CAD build for the part. Positions are in the model's coordinates, mm. Face numbers are marked on the shaded views. A direction names the side the tool comes from. Coordinates: 2 decimals unless noted, no trailing zeros. Order: outer loops, then holes, each group sorted by start corner. A loop starts at its lowest first (then second) coordinate and runs counter-clockwise, first axis right, second up. Notation, with made-up numbers: M 81.25,69.25 L 119.25,69.25 A15 ccw 119.25,96.25 Z; hole C 3.5,71.5 d9. An arc over 180 degrees is marked long. One line per item, written item: value.
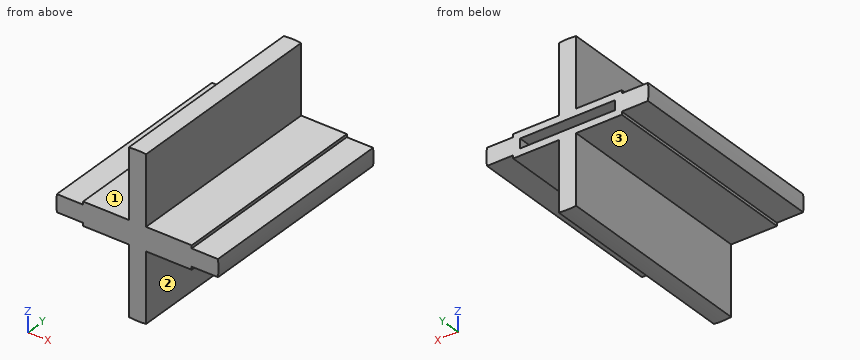
from build123d import *

# Parameters (mm, degrees)
SKETCH1_W           = 19.346272943
SKETCH1_H           = 12.7
SKETCH1_W_2         = 33.655
SKETCH1_H_2         = 2.2225
SKETCH1_W_3         = 12.7
SKETCH1_H_3         = 2.8575
SKETCH1_H_4         = 50.778772943
BOSS_EXTRUDE1_DEPTH = 76.2
SKETCH2_W           = 80.01
SKETCH2_H           = 17.145
BOSS_EXTRUDE2_DEPTH = 6.35


with BuildPart() as part:
    # Sketch1 → Boss-Extrude1 (new body, symmetric)
    with BuildSketch(Plane(origin=(0, 0, 0), x_dir=(1, 0, 0), z_dir=(0, 1, 0))):
        with Locations((-49.678136472, 0)):
            Rectangle(SKETCH1_W, SKETCH1_H)
        with BuildLine():
            ThreePointArc((-59.351272943, 6.35), (-59.69, 0), (-59.351272943, -6.35))
            Line((-59.351272943, -6.35), (-59.351272943, 6.35))
        make_face()
        with Locations((-23.1775, -7.46125)):
            Rectangle(SKETCH1_W_2, SKETCH1_H_2)
        Polygon((-6.35, -3.4925), (-34.925, -3.4925), (-34.925, 3.4925), (-6.35, 3.4925), (-6.35, 6.35), (-40.005, 6.35), (-40.005, -6.35), (-6.35, -6.35), align=None)
        with Locations((-23.1775, 7.46125)):
            Rectangle(SKETCH1_W_2, SKETCH1_H_2)
        with Locations((0, 7.46125)):
            Rectangle(SKETCH1_W_3, SKETCH1_H_2)
        with Locations((0, 4.92125)):
            Rectangle(SKETCH1_W_3, SKETCH1_H_3)
        with Locations((23.1775, 7.46125)):
            Rectangle(SKETCH1_W_2, SKETCH1_H_2)
        Polygon((34.925, -3.4925), (6.35, -3.4925), (6.35, -6.35), (40.005, -6.35), (40.005, 6.35), (6.35, 6.35), (6.35, 3.4925), (34.925, 3.4925), align=None)
        with Locations((23.1775, -7.46125)):
            Rectangle(SKETCH1_W_2, SKETCH1_H_2)
        with Locations((0, -7.46125)):
            Rectangle(SKETCH1_W_3, SKETCH1_H_2)
        with Locations((0, -4.92125)):
            Rectangle(SKETCH1_W_3, SKETCH1_H_3)
        with Locations((0, -33.961886472)):
            Rectangle(SKETCH1_W_3, SKETCH1_H_4)
        with BuildLine():
            Line((6.35, -59.351272943), (-6.35, -59.351272943))
            ThreePointArc((-6.35, -59.351272943), (0, -59.69), (6.35, -59.351272943))
        make_face()
        with Locations((49.678136472, 0)):
            Rectangle(SKETCH1_W, SKETCH1_H)
        with BuildLine():
            Line((59.351272943, 6.35), (59.351272943, -6.35))
            ThreePointArc((59.351272943, -6.35), (59.605258082, -3.179513957), (59.69, 0))
            ThreePointArc((59.69, 0), (59.605258082, 3.179513957), (59.351272943, 6.35))
        make_face()
        with Locations((0, 33.961886472)):
            Rectangle(SKETCH1_W_3, SKETCH1_H_4)
        with BuildLine():
            ThreePointArc((6.35, 59.351272943), (0, 59.69), (-6.35, 59.351272943))
            Line((-6.35, 59.351272943), (6.35, 59.351272943))
        make_face()
    extrude(amount=BOSS_EXTRUDE1_DEPTH, both=True)

    # Sketch2 → Boss-Extrude2 (add)
    with BuildSketch(Plane.XZ.offset(76.2)):
        Rectangle(SKETCH2_W, SKETCH2_H)
    extrude(amount=-BOSS_EXTRUDE2_DEPTH)


solid = part.part
Q1. Slice it at C-C (z = -26). List the corners of the cut face in (x, y), plus the area to 3 significant figures.
Recorded:
outline: M -6.35,-76.2 L 6.35,-76.2 L 6.35,76.2 L -6.35,76.2 Z
area: 1,940 mm^2
Q2. Which spindle directions (+Z, -Z, +X, -X, +Y, -Y) get a long thin tool onto all of the face, cutting with end or side? Do the marked faces 1, 2 and 3. Say none if no direction does.
Recorded:
face 1: +Z, -X, +Y, -Y
face 2: -Z, +X, +Y, -Y
face 3: -Z, -X, +Y, -Y
Q3. Slice it at B-B (x = -21). List the corners of the cut face in (y, z), plus the area to 3 significant figures.
Recorded:
outline: M -76.2,-8.57 L 76.2,-8.57 L 76.2,-3.49 L -69.85,-3.49 L -69.85,3.49 L 76.2,3.49 L 76.2,8.57 L -76.2,8.57 Z
area: 1,590 mm^2
Q4. Drill centre lines: line 1 along X through (y, z) = (-31.5, 0.5) (3 decimals); line 2 along Z through (x, y) = (25, 26); line 3 along Z through (x, y) = (2, 27). Where is each one in solid material? Low to high.
Recorded:
line 1: x = -59.688 to -34.925, 34.925 to 59.688
line 2: z = -8.57 to -3.49, 3.49 to 8.57
line 3: z = -59.66 to -3.49, 3.49 to 59.66
Q5. Pin check, flat tips, straight feed: pin 1 Ø2 at (x, y) = (47, -32.5) entering from -Z; pin 2 Ø2 at (x, y) = (-14.5, 59) entering from +Z; pin 3 Ø1.5 at (x, y) = (-30.5, 0) entering from -Z; pin 4 Ø10 at (x, z) = (-23, -18.5) entering from +Y. Stop position of each tip, or through.
Recorded:
pin 1: stops at z = -6.35
pin 2: stops at z = 8.57
pin 3: stops at z = -8.57
pin 4: passes through
Q6. Slice it at D-D (x = 44.5). List the corners of the cut face in (y, z), plus the area to 3 significant figures.
Recorded:
outline: M -76.2,-6.35 L 76.2,-6.35 L 76.2,6.35 L -76.2,6.35 Z
area: 1,940 mm^2
